from build123d import *

# Parameters (mm, degrees)
SKETCH_1_W             = 650
SKETCH_1_H             = 460
EXTRUDE_1_DEPTH        = 4
SKETCH_3_R             = 2.05
CUT_EXTRUDE_2_DEPTH    = 5
CUT_EXTRUDE_1515_DEPTH = 5
SKETCH_5_R             = 2.6
CUT_EXTRUDE_2177_DEPTH = 5
FILLET_1_R             = 80
CUT_EXTRUDE_2788_DEPTH = 5
CUT_EXTRUDE_3372_DEPTH = 5
SKETCH_8_R             = 1.5
CUT_EXTRUDE_3986_DEPTH = 5
SKETCH_9_R             = 2.25
CUT_EXTRUDE_4689_DEPTH = 5
FILLET_2_R             = 80
SKETCH_10_R            = 1.6
SKETCH_10_W            = 5
SKETCH_10_H            = 95
CUT_EXTRUDE_5264_DEPTH = 5
FILLET_3_R             = 5
FILLET_4_R             = 2
SKETCH_11_W            = 2
SKETCH_11_H            = 3
CUT_EXTRUDE_6150_DEPTH = 5
CUT_EXTRUDE_6369_DEPTH = 5
SKETCH_13_W            = 15
SKETCH_13_H            = 5
CUT_EXTRUDE_6552_DEPTH = 5
SKETCH_15_R            = 2
SKETCH_15_R_2          = 4
CUT_EXTRUDE_6861_DEPTH = 5
SKETCH_16_R            = 5
SKETCH_16_R_2          = 10
SKETCH_16_R_3          = 4
CUT_EXTRUDE_12_DEPTH   = 5
SKETCH_17_R            = 2
CUT_EXTRUDE_13_DEPTH   = 5
SKETCH_18_R            = 1.6
CUT_EXTRUDE_14_DEPTH   = 5


with BuildPart() as part:
    # 草图1 → 凸台-拉伸1 (new body)
    with BuildSketch(Plane(origin=(0, 0, 0), x_dir=(1, 0, 0), z_dir=(0, 1, 0))):
        Rectangle(SKETCH_1_W, SKETCH_1_H)
    extrude(amount=EXTRUDE_1_DEPTH)

    # 草图3 → 切除-拉伸2 (cut, through all)
    with BuildSketch(Plane(origin=(0, 4, 0), x_dir=(1, 0, 0), z_dir=(0, 1, 0))):
        with Locations((230, 165)):
            Circle(SKETCH_3_R)
        with Locations((265, 165)):
            Circle(SKETCH_3_R)
        with Locations((265, 100)):
            Circle(SKETCH_3_R)
        with Locations((230, 100)):
            Circle(SKETCH_3_R)
    extrude(amount=-CUT_EXTRUDE_2_DEPTH, mode=Mode.SUBTRACT)

    # 草图4 → Cut-Extrude 1515 (cut, through all)
    with BuildSketch(Plane(origin=(0, 4, 0), x_dir=(1, 0, 0), z_dir=(0, 1, 0))):
        Polygon((-204.791847198, 53.223304703), (-130.545635174, 127.469516728), (-17.408550184, 14.332431738), (-91.654762208, -59.913780286), align=None)
    extrude(amount=-CUT_EXTRUDE_1515_DEPTH, mode=Mode.SUBTRACT)

    # 草图5 → Cut-Extrude 2177 (cut, through all)
    with BuildSketch(Plane(origin=(0, 4, 0), x_dir=(1, 0, 0), z_dir=(0, 1, 0))):
        with Locations((165, -216)):
            Circle(SKETCH_5_R)
        with Locations((-315, -216)):
            Circle(SKETCH_5_R)
        with Locations((-315, 216)):
            Circle(SKETCH_5_R)
        with Locations((165, 216)):
            Circle(SKETCH_5_R)
        with Locations((-315, 96)):
            Circle(SKETCH_5_R)
        with Locations((-315, -96)):
            Circle(SKETCH_5_R)
    extrude(amount=-CUT_EXTRUDE_2177_DEPTH, mode=Mode.SUBTRACT)

    # 圆角1
    fillet_1_edges = [part.edges().sort_by_distance(p)[0] for p in [
        (325, 2, -230),
    ]]
    fillet(fillet_1_edges, radius=FILLET_1_R)

    # 草图6 → Cut-Extrude 2788 (cut, through all)
    with BuildSketch(Plane(origin=(0, 4, 0), x_dir=(1, 0, 0), z_dir=(0, 1, 0))):
        with BuildLine():
            Line((10, 163.6), (20, 163.6))
            ThreePointArc((20, 163.6), (21.6, 162), (20, 160.4))
            Line((20, 160.4), (10, 160.4))
            ThreePointArc((10, 160.4), (8.4, 162), (10, 163.6))
        make_face()
        with BuildLine():
            Line((88, 163.6), (98, 163.6))
            ThreePointArc((98, 163.6), (99.6, 162), (98, 160.4))
            Line((98, 160.4), (88, 160.4))
            ThreePointArc((88, 160.4), (86.4, 162), (88, 163.6))
        make_face()
    extrude(amount=-CUT_EXTRUDE_2788_DEPTH, mode=Mode.SUBTRACT)

    # 草图7 → Cut-Extrude 3372 (cut, through all)
    with BuildSketch(Plane(origin=(0, 4, 0), x_dir=(1, 0, 0), z_dir=(0, 1, 0))):
        with BuildLine():
            Line((247.1, -61), (247.1, -121))
            ThreePointArc((247.1, -121), (245, -123.1), (242.9, -121))
            Line((242.9, -121), (242.9, -61))
            ThreePointArc((242.9, -61), (245, -58.9), (247.1, -61))
        make_face()
        with BuildLine():
            Line((97.1, -61), (97.1, -121))
            ThreePointArc((97.1, -121), (95, -123.1), (92.9, -121))
            Line((92.9, -121), (92.9, -61))
            ThreePointArc((92.9, -61), (95, -58.9), (97.1, -61))
        make_face()
        with BuildLine():
            Line((-52.9, -61), (-52.9, -121))
            ThreePointArc((-52.9, -121), (-55, -123.1), (-57.1, -121))
            Line((-57.1, -121), (-57.1, -61))
            ThreePointArc((-57.1, -61), (-55, -58.9), (-52.9, -61))
        make_face()
    extrude(amount=-CUT_EXTRUDE_3372_DEPTH, mode=Mode.SUBTRACT)

    # 草图8 → Cut-Extrude 3986 (cut, through all)
    with BuildSketch(Plane(origin=(0, 4, 0), x_dir=(1, 0, 0), z_dir=(0, 1, 0))):
        with Locations((-130, 212)):
            Circle(SKETCH_8_R)
        with Locations((-72, 212)):
            Circle(SKETCH_8_R)
        with Locations((-72, 162)):
            Circle(SKETCH_8_R)
        with Locations((-130, 162)):
            Circle(SKETCH_8_R)
    extrude(amount=-CUT_EXTRUDE_3986_DEPTH, mode=Mode.SUBTRACT)

    # 草图9 → Cut-Extrude 4689 (cut, through all)
    with BuildSketch(Plane(origin=(0, 4, 0), x_dir=(1, 0, 0), z_dir=(0, 1, 0))):
        with Locations((-225, -220)):
            Circle(SKETCH_9_R)
        with Locations((-197, -220)):
            Circle(SKETCH_9_R)
        with Locations((-169, -220)):
            Circle(SKETCH_9_R)
        with Locations((-141, -220)):
            Circle(SKETCH_9_R)
        with Locations((-113, -220)):
            Circle(SKETCH_9_R)
        with Locations((-85, -220)):
            Circle(SKETCH_9_R)
        with Locations((-57, -220)):
            Circle(SKETCH_9_R)
        with Locations((-29, -220)):
            Circle(SKETCH_9_R)
        with Locations((-1, -220)):
            Circle(SKETCH_9_R)
        with Locations((27, -220)):
            Circle(SKETCH_9_R)
        with Locations((55, -220)):
            Circle(SKETCH_9_R)
        with Locations((-197, -134)):
            Circle(SKETCH_9_R)
        with Locations((-169, -134)):
            Circle(SKETCH_9_R)
        with Locations((-141, -134)):
            Circle(SKETCH_9_R)
        with Locations((-113, -134)):
            Circle(SKETCH_9_R)
        with Locations((-85, -134)):
            Circle(SKETCH_9_R)
        with Locations((-57, -134)):
            Circle(SKETCH_9_R)
        with Locations((-29, -134)):
            Circle(SKETCH_9_R)
        with Locations((-1, -134)):
            Circle(SKETCH_9_R)
        with Locations((27, -134)):
            Circle(SKETCH_9_R)
        with Locations((55, -134)):
            Circle(SKETCH_9_R)
        with Locations((-225, -134)):
            Circle(SKETCH_9_R)
    extrude(amount=-CUT_EXTRUDE_4689_DEPTH, mode=Mode.SUBTRACT)

    # 圆角2
    fillet_2_edges = [part.edges().sort_by_distance(p)[0] for p in [
        (325, 2, 230),
    ]]
    fillet(fillet_2_edges, radius=FILLET_2_R)

    # 草图10 → Cut-Extrude 5264 (cut, through all)
    with BuildSketch(Plane(origin=(0, 4, 0), x_dir=(1, 0, 0), z_dir=(0, 1, 0))):
        with Locations((115, 50)):
            Circle(SKETCH_10_R)
        with Locations((115, 0)):
            Circle(SKETCH_10_R)
        with Locations((90, 0)):
            Circle(SKETCH_10_R)
        with Locations((90, 50)):
            Circle(SKETCH_10_R)
        with Locations((47.5, 35)):
            Rectangle(SKETCH_10_W, SKETCH_10_H)
        with Locations((157.5, 35)):
            Rectangle(SKETCH_10_W, SKETCH_10_H)
    extrude(amount=-CUT_EXTRUDE_5264_DEPTH, mode=Mode.SUBTRACT)

    # 圆角3
    fillet_3_edges = [part.edges().sort_by_distance(p)[0] for p in [
        (-91.654762208, 2, 59.913780286),
        (-204.791847198, 2, -53.223304703),
        (-130.545635174, 2, -127.469516728),
        (-17.408550184, 2, -14.332431738),
    ]]
    fillet(fillet_3_edges, radius=FILLET_3_R)

    # 圆角4
    fillet_4_edges = [part.edges().sort_by_distance(p)[0] for p in [
        (155, 2, 12.5),
        (155, 2, -82.5),
        (160, 2, -82.5),
        (160, 2, 12.5),
        (50, 2, -82.5),
        (50, 2, 12.5),
        (45, 2, 12.5),
        (45, 2, -82.5),
    ]]
    fillet(fillet_4_edges, radius=FILLET_4_R)

    # 草图11 → Cut-Extrude 6150 (cut, through all)
    with BuildSketch(Plane(origin=(0, 4, 0), x_dir=(1, 0, 0), z_dir=(0, 1, 0))):
        with BuildLine():
            Line((288, -138.4), (298, -138.4))
            ThreePointArc((298, -138.4), (299.6, -140), (298, -141.6))
            Line((298, -141.6), (288, -141.6))
            ThreePointArc((288, -141.6), (286.4, -140), (288, -138.4))
        make_face()
        with Locations((293.262535805, -122)):
            Rectangle(SKETCH_11_W, SKETCH_11_H)
    extrude(amount=-CUT_EXTRUDE_6150_DEPTH, mode=Mode.SUBTRACT)

    # 草图12 → Cut-Extrude 6369 (cut, through all)
    with BuildSketch(Plane(origin=(0, 4, 0), x_dir=(1, 0, 0), z_dir=(0, 1, 0))):
        with BuildLine():
            Line((-178.911739007, 15.463802588), (-171.840671195, 8.392734776))
            ThreePointArc((-171.840671195, 8.392734776), (-171.840671195, 6.129993076), (-174.103412895, 6.129993076))
            Line((-174.103412895, 6.129993076), (-181.174480707, 13.201060888))
            ThreePointArc((-181.174480707, 13.201060888), (-181.174480707, 15.463802588), (-178.911739007, 15.463802588))
        make_face()
    extrude(amount=-CUT_EXTRUDE_6369_DEPTH, mode=Mode.SUBTRACT)

    # 草图13 → Cut-Extrude 6552 (cut, through all)
    with BuildSketch(Plane(origin=(0, 4, 0), x_dir=(1, 0, 0), z_dir=(0, 1, 0))):
        with Locations((102.5, -17.5)):
            Rectangle(SKETCH_13_W, SKETCH_13_H)
    extrude(amount=-CUT_EXTRUDE_6552_DEPTH, mode=Mode.SUBTRACT)

    # 草图15 → Cut-Extrude 6861 (cut, through all)
    with BuildSketch(Plane(origin=(0, 4, 0), x_dir=(1, 0, 0), z_dir=(0, 1, 0))):
        with Locations((-167, -40)):
            Circle(SKETCH_15_R)
        with Locations((-205, -40)):
            Circle(SKETCH_15_R_2)
    extrude(amount=-CUT_EXTRUDE_6861_DEPTH, mode=Mode.SUBTRACT)

    # 草图16 → 切除-拉伸12 (cut, through all)
    with BuildSketch(Plane(origin=(0, 4, 0), x_dir=(1, 0, 0), z_dir=(0, 1, 0))):
        with Locations((-137.616702986, -28.093975133)):
            Circle(SKETCH_16_R)
        with Locations((-295, -180)):
            Circle(SKETCH_16_R_2)
        with Locations((135.386397476, -180)):
            Circle(SKETCH_16_R_2)
        with Locations((-207.1, -91)):
            Circle(SKETCH_16_R_3)
    extrude(amount=-CUT_EXTRUDE_12_DEPTH, mode=Mode.SUBTRACT)

    # 草图17 → 切除-拉伸13 (cut, through all)
    with BuildSketch(Plane(origin=(0, 4, 0), x_dir=(1, 0, 0), z_dir=(0, 1, 0))):
        with Locations((-300, 190)):
            Circle(SKETCH_17_R)
        with Locations((-300, 180)):
            Circle(SKETCH_17_R)
    extrude(amount=-CUT_EXTRUDE_13_DEPTH, mode=Mode.SUBTRACT)

    # 草图18 → 切除-拉伸14 (cut, through all)
    with BuildSketch(Plane(origin=(0, 4, 0), x_dir=(1, 0, 0), z_dir=(0, 1, 0))):
        with Locations((-66.552471476, 134.89413793)):
            Circle(SKETCH_18_R)
        with Locations((-56.299423149, 102.720779386)):
            Circle(SKETCH_18_R)
    extrude(amount=-CUT_EXTRUDE_14_DEPTH, mode=Mode.SUBTRACT)


solid = part.part
Geometry: final body of the model. Coordinates: model frame, mm. A direction names the side the tool comes from. Round coordinates to 2 decimals unless told otherwise and drop trailing zeros. Order: outer loops, then holes, each group sorted by start corner. A loop starts at its lowest first (then second) coordinate and runs counter-clockwise, first axis right, second up.
Q1. Pin query (flat end, axial travel): pin 1 (2 mm diameter, centred on x = 294.5, y = 2, fed in from +Z); pin 2 (1.6 mm diameter, centred on x = 293, y = 1, fed in from -Z); pin 3 (1.9 mm diameter, centred on x = 90, z = -50, fed in from -Y); pin 4 (5.5 mm diameter, centred on x = 265, z = -165, fed in from +Y). Return the tip coordinate at first contact, or that it passes through.
Result sheet:
pin 1: stops at z = 213.62
pin 2: stops at z = -214.59
pin 3: passes through
pin 4: stops at y = 4
Q2. Section C-C, the plane y = 3.1. Give the number of separate pieces and of enclosed holes in the cut face, and give its area (3 significant figures).
Result sheet:
separate pieces: 1
enclosed holes: 62
area: 276,000 mm2
Q3. Material intervals for probe 1 along X at (y, z) = (1.4, 27.5); probe 2 along Z at (x, y) = (-225, 1.2); probe 3 along X at (y, z) = (0.7, 105.5), sorted ascending.
Result sheet:
probe 1: x = -325 to -142.58, -132.65 to -124.07, -59.24 to 325
probe 2: z = -230 to 131.75, 136.25 to 217.75, 222.25 to 230
probe 3: x = -325 to -57.1, -52.9 to 92.9, 97.1 to 242.9, 247.1 to 325
Q4. Access query for faces 1 (the face through (-54.06, 2.03, 22.32)), 2 (the face through (300.94, 2.03, -207.19)). Directions: +Z, -Z, +X, -X, +Y, -Y. A direction counts if a zero-diameter tool reaches every point of the face in a straight line with its end or side. Return the directions, or none.
Result sheet:
face 1: +Y, -Y
face 2: -Z, +X, +Y, -Y
Q5. Section A-A, the plane x = -158. Output: boundary loops of the cut face in (y, z), and give its area (3 significant figures).
Result sheet:
outline: (0, -230) - (4, -230) - (4, -100.02) - (0, -100.02) - close; (0, -6.43) - (4, -6.43) - (4, 230) - (0, 230) - close
area: 1,470 mm2
Q6. Mould query, pull axis X, two halves, no side actions, for faces 3 (the face through (302.19, 2.03, 205.94)), 4 (the face through (-5, 0, -3)), 5 (the face through (144.624, 2.028, 183.83)), 6 (the face through (-147.48, 2.03, 4.09)). Classes: released by +X, released by -X, zero draft, split by the parting line, or undercut.
Result sheet:
face 3: released by +X
face 4: zero draft
face 5: undercut
face 6: undercut
Q7. Section B-B, the plane z = 180. Output: boundary loops of the cut face in (x, y), and give its area (3 significant figures).
Result sheet:
outline: (-325, 0) - (-305, 0) - (-305, 4) - (-325, 4) - close; (-285, 0) - (125.39, 0) - (125.39, 4) - (-285, 4) - close; (145.39, 0) - (319.16, 0) - (319.16, 4) - (145.39, 4) - close
area: 2,420 mm2
